```python
from build123d import *

# Parameters (mm, degrees)
F0_R     = 1.27
F1_DEPTH = 2.2


with BuildPart() as f1:
    # F0 (on Top) → F1 (new body)
    with BuildSketch(Plane.XY):
        with BuildLine():
            ThreePointArc((0, 7), (2.050253, 2.050253), (7, 0))
            Line((7, 0), (27, 0))
            ThreePointArc((27, 0), (31.949747, 2.050253), (34, 7))
            Line((34, 7), (34, 19.25))
            ThreePointArc((34, 19.25), (31.949747, 24.199747), (27, 26.25))
            Line((27, 26.25), (7, 26.25))
            ThreePointArc((7, 26.25), (2.050253, 24.199747), (0, 19.25))
            Line((0, 19.25), (0, 7))
        make_face()
        with Locations((16.231103, 3.355003)):
            Circle(F0_R, mode=Mode.SUBTRACT)
        with Locations((16.231103, 23.15167)):
            Circle(F0_R, mode=Mode.SUBTRACT)
        Polygon((4.537634, 7), (4.537634, 19.25), (27, 19.25), (27, 15.8), (29.597666, 15.8), (29.597666, 10.45), (27, 10.45), (27, 7), align=None, mode=Mode.SUBTRACT)
    extrude(amount=F1_DEPTH)


solid = f1.part
```
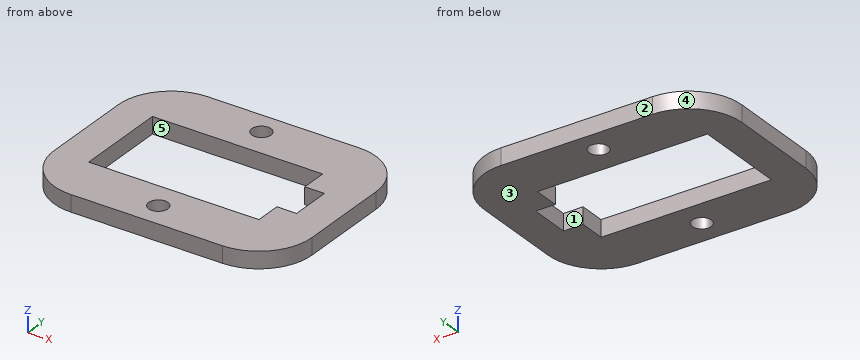
CAD build for the part. Positions are in the model's coordinates, mm. Face numbers are marked on the shaded views. A direction names the side the tool comes from. Round coordinates to 2 decimals unless told otherwise and drop trailing zeros. Write each loop counter-clockwise with the first axis right and the second up, starting at its lowest first coordinate (ties: lowest second). Pieces come first, ordered by that corner, then holes.
Item 1: Drop flat-ended pins along their axis: pin 1 Ø0.7 at (x, z) = (28, 1) entering from +Y; pin 2 Ø1 at (y, z) = (22, 0.5) entering from +X. Give the stop position or say it passes through.
Filled in:
pin 1: stops at y = 26.22
pin 2: stops at x = 33.63
Item 2: Drill centre lines: L1, parallel to X at y = 9.5, z = 0.9; L2, parallel to Y at x = 10, z = 0.2; L3, parallel to X at y = 12, z = 0.25. Where is each one in solid material? Low to high.
Filled in:
L1: x = 0 to 4.54, 27 to 34
L2: y = 0 to 7, 19.25 to 26.25
L3: x = 0 to 4.54, 29.6 to 34
Item 3: Band-saw the part on C-C on z = 1.25. Write the cut outline in (x, y) (3 decimals).
Filled in:
outline: (0, 7) arc R7 ccw to (7, 0) - (27, 0) arc R7 ccw to (34, 7) - (34, 19.25) arc R7 ccw to (27, 26.25) - (7, 26.25) arc R7 ccw to (0, 19.25) - close; hole (4.538, 7) - (27, 7) - (27, 10.45) - (29.598, 10.45) - (29.598, 15.8) - (27, 15.8) - (27, 19.25) - (4.538, 19.25) - close; hole circle Ø2.54 at (16.231, 3.355); hole circle Ø2.54 at (16.231, 23.152)
Item 4: Mould opens along X. For the marked faces 3, 4 and 5 say: released by +X, released by -X, zero draft, split by the parting line, or undercut.
Filled in:
face 3: zero draft
face 4: released by -X
face 5: undercut
Item 5: Tool access for the marked faces 1 and 2: list every direction of +Z, -Z, +X, -X, +Y, -Y with a clear straight run to the whole face (end or side of a thin tool).
Filled in:
face 1: +Z, -Z
face 2: +Z, -Z, +X, -X, +Y
Item 6: Band-saw the part on A-A on y = 13. Write the cut outline in (x, z), then the cut area to 3 significant figures.
Filled in:
outline: (0, 0) - (4.54, 0) - (4.54, 2.2) - (0, 2.2) - close; (29.6, 0) - (34, 0) - (34, 2.2) - (29.6, 2.2) - close
area: 19.7 mm2
Item 7: Band-saw the part on B-B on x = 14.5. Write the cut outline in (y, z).
Filled in:
outline: (0, 0) - (7, 0) - (7, 2.2) - (0, 2.2) - close; (19.25, 0) - (26.25, 0) - (26.25, 2.2) - (19.25, 2.2) - close
Item 8: Band-saw the part on D-D on y = 5. Write the cut outline in (x, z), then the cut area to 3 significant figures.
Filled in:
outline: (0.29, 0) - (33.71, 0) - (33.71, 2.2) - (0.29, 2.2) - close
area: 73.5 mm2
